Read the model definition and answer for the solid it produces. Units are mm, in the model's axes. A direction names the side the tool comes from. Coordinates: 2 decimals unless noted, no trailing zeros. Order: outer loops, then holes, each group sorted by start corner. A loop starts at its lowest first (then second) coordinate and runs counter-clockwise, first axis right, second up. Notation, with made-up numbers: M 29,-2 L 76,-2 A28 ccw 76,29 Z; hole C -4,-34.5 d5. An arc over 180 degrees is marked long. Put each result on its own line as item: value.
from build123d import *

# Parameters (mm, degrees)
SKETCH1_R               = 5.5
BOSS_EXTRUDE1_DEPTH     = 35
SKETCH2_R               = 7.5
BOSS_EXTRUDE2_DEPTH     = 5
SKETCH3_R               = 1
CUT_EXTRUDE1_DEPTH      = 8.5
CUT_EXTRUDE1_DEPTH_BACK = 8.5


with BuildPart() as part:
    # Sketch1 → Boss-Extrude1 (new body)
    with BuildSketch(Plane(origin=(0, 0, 0), x_dir=(0, 0, -1), z_dir=(1, 0, 0))):
        Circle(SKETCH1_R)
    extrude(amount=-BOSS_EXTRUDE1_DEPTH)

    # Sketch2 → Boss-Extrude2 (add)
    with BuildSketch(Plane.ZY.offset(35)):
        Circle(SKETCH2_R)
    extrude(amount=BOSS_EXTRUDE2_DEPTH)

    # Sketch3 → Cut-Extrude1 (cut, two sides)
    with BuildSketch(Plane.XY) as cut_extrude1_sk:
        with Locations((-4, 0)):
            Circle(SKETCH3_R)
    extrude(amount=CUT_EXTRUDE1_DEPTH, mode=Mode.SUBTRACT)
    extrude(cut_extrude1_sk.sketch, amount=-CUT_EXTRUDE1_DEPTH_BACK, mode=Mode.SUBTRACT)


solid = part.part
Q1. Find section D-D on x = -32. Write down the section's boundary in (y, z), plus the area to 3 significant figures.
Answers below:
outline: C 0,0 d11
area: 95.0 mm^2
Q2. Consider line 1 along X through (y, z) = (0, 3); line 2 along Y through (x, z) = (-4, -1.75); line 3 along Y through (x, z) = (-29, 0.25). Determine where each line is inside the solid, lowest interval first.
Answers below:
line 1: x = -40 to -5, -3 to 0
line 2: y = -5.21 to -1, 1 to 5.21
line 3: y = -5.49 to 5.49
Q3. Find section B-B on z = 0. Write down the section's boundary in (x, y), plus the area to 3 significant figures.
Answers below:
outline: M -40,-7.5 L -35,-7.5 L -35,-5.5 L 0,-5.5 L 0,5.5 L -35,5.5 L -35,7.5 L -40,7.5 Z; hole C -4,0 d2
area: 457 mm^2
Q4. Given pin 1 (8 mm diameter, centred on x = -7, z = 0.5, fed in from -Y); pin 2 (5 mm diameter, centred on x = -15.5, y = -1, fed in from -Z); pin 3 (5 mm diameter, centred on x = -5, z = -0.5, fed in from +Y), each flat-ended and moving along its own axis, determine where each tip first touches the part or whether it passes through.
Answers below:
pin 1: stops at y = -5.5
pin 2: stops at z = -5.5
pin 3: stops at y = 5.5
Q5. A tool of negligible diameter and unlimited length cuts with its end or side. For faces 1 (the face through (-4.8, -0.6, 0.1)), 2 (the face through (-17.26, -5.37, 1.19)), from which of +Z, -Z, +X, -X, +Y, -Y can it reach the whole face along a straight path? Write none if from no direction.
Answers below:
face 1: +Z, -Z
face 2: +X
Q6. For a pull along Z with two mould halves and no side action, classify faces 3 (the face through (0, 0, 0)), 4 (the face through (-37.465, 0.33, -7.493)) as +Z half, -Z half, draft (parallel to the pull), parting line (faces both ways), or undercut.
Answers below:
face 3: draft
face 4: parting line
Q7. Find section A-A on y = 0. Write down the section's boundary in (x, z).
Answers below:
outline: M -40,-7.5 L -35,-7.5 L -35,-5.5 L -5,-5.5 L -5,5.5 L -35,5.5 L -35,7.5 L -40,7.5 Z; M -3,-5.5 L 0,-5.5 L 0,5.5 L -3,5.5 Z
Q8. Find section C-C on y = -4.75. Write down the section's boundary in (x, z).
Answers below:
outline: M -40,-5.8 L -35,-5.8 L -35,-2.77 L 0,-2.77 L 0,2.77 L -35,2.77 L -35,5.8 L -40,5.8 Z
